Source: CAD feature listing. Evaluate the final solid. Frame: model axes, mm. A direction names the side the tool comes from. Give positions to 0.01 mm unless a question says otherwise; leave off trailing zeros. Order: outer loops, then holes, each group sorted by start corner. A loop starts at its lowest first (then second) coordinate and runs counter-clockwise, first axis right, second up.
from build123d import *

# Parameters (mm, degrees)
SKETCH1_W            = 70
SKETCH1_H            = 20
SKETCH1_W_2          = 264.8
EXTRUDE_1017_DEPTH   = 8
SKETCH2_W            = 36
SKETCH2_H            = 8
BOSS_EXTRUDE2_DEPTH  = 8
SKETCH4_W            = 36
SKETCH4_H            = 8
BOSS_EXTRUDE3_DEPTH  = 8
SKETCH5_R            = 1.5
CUT_EXTRUDE1_DEPTH   = 349.438631613
FILLET1_R            = 2.5
SKETCH6_W            = 52
SKETCH6_H            = 20
CUT_EXTRUDE2_DEPTH   = 349.438631613
SKETCH7_W            = 16.8
SKETCH7_H            = 20
CUT_EXTRUDE3_DEPTH   = 299.821485171
SKETCH8_W            = 30
SKETCH8_H            = 8
BOSS_EXTRUDE4_DEPTH  = 30
SKETCH9_W            = 30
SKETCH9_H            = 8
BOSS_EXTRUDE5_DEPTH  = 30
SKETCH10_W           = 8
SKETCH10_H           = 50
CUT_EXTRUDE4_DEPTH   = 307.61226329
SKETCH12_W           = 11
SKETCH12_H           = 50
BOSS_EXTRUDE6_DEPTH  = 17
SKETCH13_W           = 8
SKETCH13_H           = 15
BOSS_EXTRUDE7_DEPTH  = 17
SKETCH15_W           = 11
SKETCH15_H           = 45
CUT_EXTRUDE6_DEPTH   = 20
SKETCH16_W           = 22
SKETCH16_H           = 8
BOSS_EXTRUDE9_DEPTH  = 5
SKETCH18_W           = 13
SKETCH18_H           = 40
BOSS_EXTRUDE10_DEPTH = 10
SKETCH21_W           = 13
SKETCH21_H           = 5
CUT_EXTRUDE9_DEPTH   = 10
SKETCH17_W           = 16
SKETCH17_H           = 22
CUT_EXTRUDE7_DEPTH   = 12
SKETCH19_W           = 70
SKETCH19_H           = 20
BOSS_EXTRUDE11_DEPTH = 17
SKETCH20_W           = 65
SKETCH20_H           = 15
CUT_EXTRUDE8_DEPTH   = 20
SKETCH22_W           = 20
SKETCH22_H           = 17
BOSS_EXTRUDE12_DEPTH = 3
BOSS_EXTRUDE13_DEPTH = 3
SKETCH24_R           = 1.65
CUT_EXTRUDE10_DEPTH  = 308.159697877
BOSS_EXTRUDE14_DEPTH = 1
FILLET4_R            = 5
FILLET5_R            = 5
FILLET7_R            = 5
FILLET8_R            = 5
FILLET9_R            = 5
FILLET10_R           = 5
FILLET11_R           = 5
FILLET12_R           = 5
FILLET13_R           = 5
FILLET14_R           = 2.5
FILLET15_R           = 2.5
FILLET16_R           = 2.5
FILLET17_R           = 5
SKETCH26_W           = 76
SKETCH26_H           = 20
BOSS_EXTRUDE15_DEPTH = 3
FILLET18_R           = 3
SKETCH27_W           = 9
SKETCH27_H           = 20
BOSS_EXTRUDE16_DEPTH = 2
FILLET20_R           = 2


with BuildPart() as part:
    # Sketch1 → Extrude 1017 (new body)
    with BuildSketch(Plane(origin=(0, 0, 0), x_dir=(1, 0, 0), z_dir=(0, 1, 0))):
        with Locations((-35, -78.2)):
            Rectangle(SKETCH1_W, SKETCH1_H)
        with Locations((132.4, -78.2)):
            Rectangle(SKETCH1_W_2, SKETCH1_H)
        with Locations((299.8, -78.2)):
            Rectangle(SKETCH1_W, SKETCH1_H)
    extrude(amount=EXTRUDE_1017_DEPTH)

    # Sketch2 → Boss-Extrude2 (add)
    with BuildSketch(Plane(origin=(0, 0, 68.2), x_dir=(-1, 0, 0), z_dir=(0, 0, -1))):
        with Locations((35.2, 4)):
            Rectangle(SKETCH2_W, SKETCH2_H)
        with Locations((-264.8, 4)):
            Rectangle(SKETCH2_W, SKETCH2_H)
    extrude(amount=BOSS_EXTRUDE2_DEPTH)

    # Sketch4 → Boss-Extrude3 (add)
    with BuildSketch(Plane.XY.offset(88.2)):
        with Locations((-35.2, 4)):
            Rectangle(SKETCH4_W, SKETCH4_H)
        with Locations((264.8, 4)):
            Rectangle(SKETCH4_W, SKETCH4_H)
    extrude(amount=BOSS_EXTRUDE3_DEPTH)

    # Sketch5 → Cut-Extrude1 (cut, through all)
    with BuildSketch(Plane(origin=(0, 8, 0), x_dir=(1, 0, 0), z_dir=(0, 1, 0))):
        with Locations(Location((-48.6, -91.6, 0), (0, 0, 270))):
            Circle(SKETCH5_R)
        with Locations(Location((-21.8, -91.6, 0), (0, 0, 270))):
            Circle(SKETCH5_R)
        with Locations(Location((-21.8, -64.8, 0), (0, 0, 270))):
            Circle(SKETCH5_R)
        with Locations(Location((-48.6, -64.8, 0), (0, 0, 270))):
            Circle(SKETCH5_R)
        with Locations(Location((278.2, -91.6, 0), (0, 0, 270))):
            Circle(SKETCH5_R)
        with Locations(Location((251.4, -64.8, 0), (0, 0, 270))):
            Circle(SKETCH5_R)
        with Locations(Location((278.2, -64.8, 0), (0, 0, 270))):
            Circle(SKETCH5_R)
        with Locations(Location((251.4, -91.6, 0), (0, 0, 270))):
            Circle(SKETCH5_R)
    extrude(amount=-CUT_EXTRUDE1_DEPTH, mode=Mode.SUBTRACT)

    # Fillet1
    fillet1_edges = [part.edges().sort_by_distance(p)[0] for p in [
        (-53.2, 4, 60.2),
        (-17.2, 4, 60.2),
        (282.8, 4, 60.2),
        (-17.2, 4, 96.2),
        (-53.2, 4, 96.2),
        (282.8, 4, 96.2),
    ]]
    fillet(fillet1_edges, radius=FILLET1_R)

    # Sketch6 → Cut-Extrude2 (cut, through all)
    with BuildSketch(Plane(origin=(0, 8, 0), x_dir=(1, 0, 0), z_dir=(0, 1, 0))):
        with Locations((308.8, -78.2)):
            Rectangle(SKETCH6_W, SKETCH6_H)
    extrude(amount=-CUT_EXTRUDE2_DEPTH, mode=Mode.SUBTRACT)

    # Sketch7 → Cut-Extrude3 (cut, through all)
    with BuildSketch(Plane(origin=(0, 0, 0), x_dir=(-1, 0, 0), z_dir=(0, -1, 0))):
        with Locations((61.6, -78.2)):
            Rectangle(SKETCH7_W, SKETCH7_H)
    extrude(amount=-CUT_EXTRUDE3_DEPTH, mode=Mode.SUBTRACT)

    # Sketch8 → Boss-Extrude4 (add)
    with BuildSketch(Plane.XY.offset(88.2)):
        with Locations((231.8, 4)):
            Rectangle(SKETCH8_W, SKETCH8_H)
    extrude(amount=BOSS_EXTRUDE4_DEPTH)

    # Sketch9 → Boss-Extrude5 (add)
    with BuildSketch(Plane(origin=(0, 0, 68.2), x_dir=(-1, 0, 0), z_dir=(0, 0, -1))):
        with Locations((-231.8, 4)):
            Rectangle(SKETCH9_W, SKETCH9_H)
    extrude(amount=BOSS_EXTRUDE5_DEPTH)

    # Sketch10 → Cut-Extrude4 (cut, through all)
    with BuildSketch(Plane(origin=(0, 0, 0), x_dir=(-1, 0, 0), z_dir=(0, -1, 0))):
        with Locations((-231.8, -78.2)):
            Rectangle(SKETCH10_W, SKETCH10_H)
    extrude(amount=-CUT_EXTRUDE4_DEPTH, mode=Mode.SUBTRACT)

    # Sketch12 → Boss-Extrude6 (add)
    with BuildSketch(Plane(origin=(0, 8, 0), x_dir=(1, 0, 0), z_dir=(0, 1, 0))):
        with Locations((222.3, -93.2)):
            Rectangle(SKETCH12_W, SKETCH12_H)
    extrude(amount=BOSS_EXTRUDE6_DEPTH)

    # Sketch13 → Boss-Extrude7 (add)
    with BuildSketch(Plane(origin=(0, 8, 0), x_dir=(1, 0, 0), z_dir=(0, 1, 0))):
        with Locations((231.8, -110.7)):
            Rectangle(SKETCH13_W, SKETCH13_H)
    extrude(amount=BOSS_EXTRUDE7_DEPTH)

    # Sketch15 → Cut-Extrude6 (cut)
    with BuildSketch(Plane(origin=(0, 0, 0), x_dir=(-1, 0, 0), z_dir=(0, -1, 0))):
        with Locations((-222.3, -95.7)):
            Rectangle(SKETCH15_W, SKETCH15_H)
    extrude(amount=-CUT_EXTRUDE6_DEPTH, mode=Mode.SUBTRACT)

    # Sketch16 → Boss-Extrude9 (add)
    with BuildSketch(Plane(origin=(246.8, 0, 0), x_dir=(0, 0, -1), z_dir=(1, 0, 0))):
        with Locations((-107.2, 4)):
            Rectangle(SKETCH16_W, SKETCH16_H)
    extrude(amount=BOSS_EXTRUDE9_DEPTH)

    # Sketch18 → Boss-Extrude10 (add)
    with BuildSketch(Plane(origin=(0, 8, 0), x_dir=(1, 0, 0), z_dir=(0, 1, 0))):
        with Locations((242.3, -98.2)):
            Rectangle(SKETCH18_W, SKETCH18_H)
    extrude(amount=BOSS_EXTRUDE10_DEPTH)

    # Sketch21 → Cut-Extrude9 (cut)
    with BuildSketch(Plane(origin=(0, 18, 0), x_dir=(1, 0, 0), z_dir=(0, 1, 0))):
        with Locations((242.3, -80.7)):
            Rectangle(SKETCH21_W, SKETCH21_H)
    extrude(amount=-CUT_EXTRUDE9_DEPTH, mode=Mode.SUBTRACT)

    # Sketch17 → Cut-Extrude7 (cut)
    with BuildSketch(Plane(origin=(0, 0, 0), x_dir=(-1, 0, 0), z_dir=(0, -1, 0))):
        with Locations((-235.8, -99.2)):
            Rectangle(SKETCH17_W, SKETCH17_H)
    extrude(amount=-CUT_EXTRUDE7_DEPTH, mode=Mode.SUBTRACT)

    # Sketch19 → Boss-Extrude11 (add)
    with BuildSketch(Plane(origin=(0, 8, 0), x_dir=(1, 0, 0), z_dir=(0, 1, 0))):
        with Locations((181.8, -78.2)):
            Rectangle(SKETCH19_W, SKETCH19_H)
    extrude(amount=BOSS_EXTRUDE11_DEPTH)

    # Sketch20 → Cut-Extrude8 (cut)
    with BuildSketch(Plane(origin=(0, 0, 0), x_dir=(-1, 0, 0), z_dir=(0, -1, 0))):
        with Locations((-184.3, -80.7)):
            Rectangle(SKETCH20_W, SKETCH20_H)
    extrude(amount=-CUT_EXTRUDE8_DEPTH, mode=Mode.SUBTRACT)

    # Sketch22 → Boss-Extrude12 (add)
    with BuildSketch(Plane.ZY.offset(-146.8)):
        with Locations((78.2, 16.5)):
            Rectangle(SKETCH22_W, SKETCH22_H)
    extrude(amount=BOSS_EXTRUDE12_DEPTH)

    # Sketch23 → Boss-Extrude13 (add)
    with BuildSketch(Plane(origin=(0, 25, 0), x_dir=(1, 0, 0), z_dir=(0, 1, 0))):
        Polygon((143.8, -68.2), (143.8, -88.2), (216.8, -88.2), (216.8, -118.2), (235.8, -118.2), (235.8, -103.2), (227.8, -103.2), (227.8, -68.2), align=None)
    extrude(amount=BOSS_EXTRUDE13_DEPTH)

    # Sketch24 → Cut-Extrude10 (cut, through all)
    with BuildSketch(Plane(origin=(0, 20, 0), x_dir=(-1, 0, 0), z_dir=(0, -1, 0))):
        with Locations(Location((-222.8, -114.2, 0), (0, 0, 90))):
            Circle(SKETCH24_R)
        with Locations(Location((-222.8, -82.2, 0), (0, 0, 90))):
            Circle(SKETCH24_R)
    extrude(amount=-CUT_EXTRUDE10_DEPTH, mode=Mode.SUBTRACT)

    # Sketch25 → Boss-Extrude14 (add)
    with BuildSketch(Plane.ZY.offset(-227.8)):
        Polygon((103.2, 20), (103.2, 12), (110.2, 12), (110.2, 0), (118.2, 0), (118.2, 20), align=None)
    extrude(amount=BOSS_EXTRUDE14_DEPTH)

    # Fillet4
    fillet4_edges = [part.edges().sort_by_distance(p)[0] for p in [
        (143.8, 8, 78.2),
    ]]
    fillet(fillet4_edges, radius=FILLET4_R)

    # Fillet5
    fillet5_edges = [part.edges().sort_by_distance(p)[0] for p in [
        (143.8, 28, 78.2),
    ]]
    fillet(fillet5_edges, radius=FILLET5_R)

    # Fillet7
    fillet7_edges = [part.edges().sort_by_distance(p)[0] for p in [
        (222.3, 8, 68.2),
    ]]
    fillet(fillet7_edges, radius=FILLET7_R)

    # Fillet8
    fillet8_edges = [part.edges().sort_by_distance(p)[0] for p in [
        (235.8, 18, 110.7),
    ]]
    fillet(fillet8_edges, radius=FILLET8_R)

    # Fillet9
    fillet9_edges = [part.edges().sort_by_distance(p)[0] for p in [
        (235.8, 28, 110.7),
    ]]
    fillet(fillet9_edges, radius=FILLET9_R - 0.0001)  # a hair under: the kernel refuses the full size

    # Fillet10
    fillet10_edges = [part.edges().sort_by_distance(p)[0] for p in [
        (216.8, 6.5, 68.2),
    ]]
    fillet(fillet10_edges, radius=FILLET10_R)

    # Fillet11
    fillet11_edges = [part.edges().sort_by_distance(p)[0] for p in [
        (242.3, 8, 83.2),
    ]]
    fillet(fillet11_edges, radius=FILLET11_R)

    # Fillet12
    fillet12_edges = [part.edges().sort_by_distance(p)[0] for p in [
        (242.3, 18, 83.2),
    ]]
    fillet(fillet12_edges, radius=FILLET12_R - 0.0001)  # a hair under: the kernel refuses the full size

    # Fillet13
    fillet13_edges = [part.edges().sort_by_distance(p)[0] for p in [
        (216.8, 24, 88.2),
    ]]
    fillet(fillet13_edges, radius=FILLET13_R)

    # Fillet14
    fillet14_edges = [part.edges().sort_by_distance(p)[0] for p in [
        (246.8, 4, 38.2),
        (216.8, 4, 38.2),
    ]]
    fillet(fillet14_edges, radius=FILLET14_R)

    # Fillet15
    fillet15_edges = [part.edges().sort_by_distance(p)[0] for p in [
        (216.8, 24, 118.2),
        (251.8, 4, 118.2),
    ]]
    fillet(fillet15_edges, radius=FILLET15_R)

    # Fillet16
    fillet16_edges = [part.edges().sort_by_distance(p)[0] for p in [
        (248.8, 13, 118.2),
    ]]
    fillet(fillet16_edges, radius=FILLET16_R)

    # Fillet17
    fillet17_edges = [part.edges().sort_by_distance(p)[0] for p in [
        (238.3, 18, 103.2),
    ]]
    fillet(fillet17_edges, radius=FILLET17_R - 0.0001)  # a hair under: the kernel refuses the full size

    # Sketch26 → Boss-Extrude15 (add)
    with BuildSketch(Plane.XY.offset(73.2)):
        with Locations((189.8, 10)):
            Rectangle(SKETCH26_W, SKETCH26_H)
    extrude(amount=BOSS_EXTRUDE15_DEPTH)

    # Fillet18
    fillet18_edges = [part.edges().sort_by_distance(p)[0] for p in [
        (151.8, 20, 82.2),
    ]]
    fillet(fillet18_edges, radius=FILLET18_R)

    # Sketch27 → Boss-Extrude16 (add)
    with BuildSketch(Plane.XY.offset(76.2)):
        with Locations((223.3, 10)):
            Rectangle(SKETCH27_W, SKETCH27_H)
    extrude(amount=BOSS_EXTRUDE16_DEPTH)

    # Fillet20
    fillet20_edges = [part.edges().sort_by_distance(p)[0] for p in [
        (151.8, 8.5, 76.2),
        (152.678679656, 19.121320344, 76.2),
        (186.8, 20, 76.2),
    ]]
    fillet(fillet20_edges, radius=FILLET20_R)


solid = part.part
1) Ray query, L1, parallel to X at y = 5, z = 91.6; L2, parallel to Z at x = 278.2, y = 5.5; L3, parallel to X at y = 2, z = 84.5. Return the intervals inside material, ascending.
Checks:
L1: x = -53.2 to -50.1, -47.1 to -23.3, -20.3 to -17.2, 243.8 to 249.9, 252.9 to 276.7, 279.7 to 282.8
L2: z = 60.2 to 63.3, 66.3 to 90.1, 93.1 to 96.2
L3: x = -53.2 to 151.8, 235.8 to 282.8
2) Reachability of faces 1 (the face through (-35, 4, 60.2)), 2 (the face through (186, 9, 76.2)), 3 (the face through (143.8, 18, 78)) from +Z, -Z, +X, -X, +Y, -Y: full face, straight path, thin tool, end or side. Return the list, or none.
Checks:
face 1: -Z, -X, +Y, -Y
face 2: +Z, -Y
face 3: +Z, -Z, -X, +Y
3) Section query B-B on y = 5. State how many separate pieces and enclosed holes the cut face has, and give its area (3 significant figures).
Checks:
separate pieces: 1
enclosed holes: 8
area: 7,870 mm2
4) Pull-direction query (X, two-part tool) for faces 4 (the face through (266, 4, 96.2)), 5 (the face through (134.2, 7.6, 68.2)), 6 (the face through (223, 10, 78.2)), 7 (the face through (-53.2, 4, 78)); classes: +X half, -X half, draft (parallel to the pull), parting line (faces both ways), or undercut.
Checks:
face 4: draft
face 5: undercut
face 6: undercut
face 7: -X half
5) First-contact query: pin 1 Ø3.5 at (x, z) = (-21.8, 91.6) entering from +Y; pin 2 Ø5 at (x, y) = (139.5, 10.5) entering from +Z; pin 3 Ø6.5 at (y, z) = (2.5, 53) entering from -X. Flat tips, straight axial feed; report the tip coordinate or a pass-through.
Checks:
pin 1: stops at y = 8
pin 2: stops at z = 88.2
pin 3: stops at x = 216.8
6) Section query A-A on x = 132. Output: boundary loops of the cut face in (y, z), and give its area (3 significant figures).
Checks:
outline: (0, 68.2) - (8, 68.2) - (8, 88.2) - (0, 88.2) - close
area: 160 mm2
